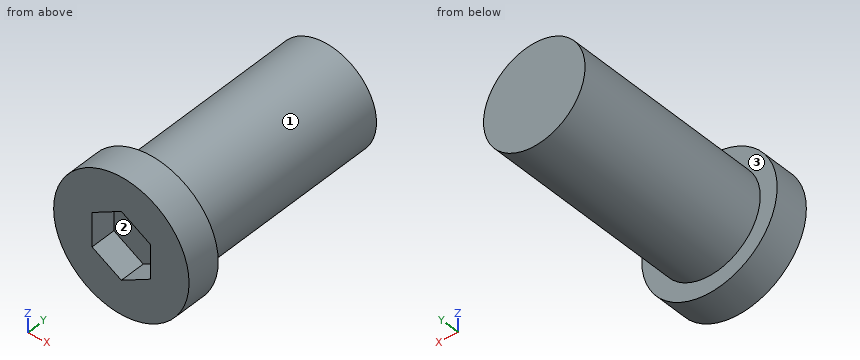
Autodesk Inventor part; units mm, degrees
ref_plane "YZ Plane" through (0, 0, 0) normal (1, 0, 0) x (0, 1, 0)
ref_plane "XZ Plane" through (0, 0, 0) normal (0, 1, 0) x (-1, 0, 0)
ref_plane "XY Plane" through (0, 0, 0) normal (0, 0, 1) x (1, 0, 0)
sketch "Sketch1" plane through (0, 0, 0) normal (0, 1, 0) x (-1, 0, 0)
  circle A0 centre (0, 0) radius 1.5
  dimension "d0" = 3
extrude "Extrusion1" add sketch "Sketch1" along normal blind 6
thread "Thread1"
sketch "Sketch2" plane through (0, 0, 0) normal (0, -1, 0) x (1, 0, 0)
  circle A0 centre (0, 0) radius 2
  dimension "d5" = 4
extrude "Extrusion2" add sketch "Sketch2" along normal blind 1
sketch "Sketch3" plane through (0, -1, 0) normal (0, -1, 0) x (1, 0, 0)
  circle A0 centre (0, 0) radius 1.5
  line L0 (0, 0) -> (0, 1)
  line L1 (0, 1) -> (0.866, 0.5)
  line L2 (0.866, 0.5) -> (0.866, -0.5)
  line L3 (0.866, -0.5) -> (0, -1)
  line L4 (0, -1) -> (-0.866, -0.5)
  line L5 (-0.866, -0.5) -> (-0.866, 0.5)
  line L6 (-0.866, 0.5) -> (0, 1)
  dimension "d8" = 1
extrude "Extrusion3" cut sketch "Sketch3" against normal blind 0.75 contours L1 L2 L3 L4 L5 L6
properties part number "Connector_2" material "Steel, Mild"
Here's how the part is built. I have some questions about the finished solid (model axes, mm). Face numbers are marked on the shaded views. Coordinates: 2 decimals unless noted, no trailing zeros. Write each loop counter-clockwise with the first axis right and the second up, starting at its lowest first coordinate (ties: lowest second). Pieces come first, ordered by that corner, then holes. Notation, with made-up numbers: (45, -32.75) - (104, -32.75) arc R27 cw to (104, -6.75) - close; hole circle Ø7 at (-17.75, 75.5). An arc over 180 degrees is marked (long way). One line per item, written item: value.
1) Suppose I cut it at C-C on x = -0.3. Write out the boundary of the cut face in (y, z).
Model answer:
outline: (-1, -1.98) - (0, -1.98) - (0, -1.47) - (6, -1.47) - (6, 1.47) - (0, 1.47) - (0, 1.98) - (-1, 1.98) - (-1, 0.83) - (-0.25, 0.83) - (-0.25, -0.83) - (-1, -0.83) - close
2) We'd pull the mould along X, two halves only. Please class the marked faces 1, 2 and 3: pulls with the +X half, pulls with the -X half, needs draft (parallel to the pull), parting line crosses it, or undercut.
Model answer:
face 1: parting line crosses it
face 2: undercut
face 3: needs draft
3) Suppose I cut it at A-A on z = -1.2. Write out the boundary of the cut face in (x, y).
Model answer:
outline: (-1.6, -1) - (1.6, -1) - (1.6, 0) - (0.9, 0) - (0.9, 6) - (-0.9, 6) - (-0.9, 0) - (-1.6, 0) - close
4) Suppose I cut it at B-B on y = 1. Write out the boundary of the cut face in (x, z).
Model answer:
outline: circle Ø3 at (0, 0)
5) I'm going to push flat-ended pins straight in: P1, Ø0.5, axis at x = 0, z = 0.5, coming from the -Y side; P2, Ø1, axis at x = 1, y = 3, coming from the +Z side. Where does each tip first touch, or does it pass through?
Model answer:
P1: stops at y = -0.25
P2: stops at z = 1.41
6) I need wall thicknesses on line 1 along Y through (x, z) = (-1.45, 0.55); line 2 along Y through (x, z) = (-0.65, -0.3); line 3 along Z through (x, y) = (-0.9, 1.5). Which ranges of each line are inside material? Lowest first, please.
Model answer:
line 1: y = -1 to 0
line 2: y = -0.25 to 6
line 3: z = -1.2 to 1.2
7) Suppose I cut it at D-D on z = 0. Write out the boundary of the cut face in (x, y).
Model answer:
outline: (-2, -1) - (-0.87, -1) - (-0.87, -0.25) - (0.87, -0.25) - (0.87, -1) - (2, -1) - (2, 0) - (1.5, 0) - (1.5, 6) - (-1.5, 6) - (-1.5, 0) - (-2, 0) - close
